Part model, mm, in its own coordinate system. A direction names the side the tool comes from. Round coordinates to 2 decimals unless told otherwise and drop trailing zeros. Loops run counter-clockwise (first coordinate to the right, second up) from the corner with the lowest first, then second, coordinate; pieces in that order, holes last.
from build123d import *

# Parameters (mm, degrees)
SKETCH1_R               = 50.00602605
SKETCH1_R_2             = 48.00602605
BOSS_EXTRUDE1_DEPTH     = 6.45
EXTRUDE_THIN1_START     = 4.55
SKETCH2_R               = 14.85
SKETCH2_R_2             = 11.85
EXTRUDE_THIN1_DEPTH     = 6.5
BOSS_EXTRUDE2_DEPTH     = 6.45
CUT_EXTRUDE1_DEPTH      = 7.45
CUT_EXTRUDE2_DEPTH      = 7.5
CUT_EXTRUDE3_DEPTH      = 1
CUT_EXTRUDE3_DEPTH_BACK = 7.5


with BuildPart() as part:
    # Sketch1 → Boss-Extrude1 (new body)
    with BuildSketch(Plane(origin=(0, 13.433589084, 0), x_dir=(-1, 0, 0), z_dir=(0, -1, 0))):
        with Locations((-83.776404782, 38.885320672)):
            Circle(SKETCH1_R)
        with Locations((-83.776404782, 38.885320672)):
            Circle(SKETCH1_R_2, mode=Mode.SUBTRACT)
    extrude(amount=BOSS_EXTRUDE1_DEPTH)



with BuildPart() as body_2:
    # Sketch2 → Extrude-Thin1 (new body)
    with BuildSketch(Plane(origin=(0, 17.983589084, 0), x_dir=(-1, 0, 0), z_dir=(0, -1, 0)).offset(EXTRUDE_THIN1_START)):
        with Locations((-208.585951979, 38.885320672)):
            Circle(SKETCH2_R)
        with Locations((-208.585951979, 38.885320672)):
            Circle(SKETCH2_R_2, mode=Mode.SUBTRACT)
    extrude(amount=EXTRUDE_THIN1_DEPTH)


with BuildPart() as part_1:
    add(part.part)

    add(body_2.part)  # Boss-Extrude2 merges body 2
    # Sketch3 → Boss-Extrude2 (add)
    with BuildSketch(Plane(origin=(0, 6.983589084, 0), x_dir=(-1, 0, 0), z_dir=(0, -1, 0))):
        with BuildLine():
            Line((-97.861971102, 86.866561409), (-212.768861048, 53.134031902))
            ThreePointArc((-212.768861048, 53.134031902), (-208.023442769, 53.724663089), (-203.336355819, 52.776477576))
            Line((-203.336355819, 52.776477576), (-113.385956141, 79.182679265))
            ThreePointArc((-113.385956141, 79.182679265), (-105.95919853, 83.701905803), (-97.861971102, 86.866561409))
        make_face()
        with BuildLine():
            Line((-113.385956141, -1.412037922), (-203.336355819, 24.994163767))
            ThreePointArc((-203.336355819, 24.994163767), (-208.023442769, 24.045978254), (-212.768861048, 24.636609441))
            Line((-212.768861048, 24.636609441), (-97.861971102, -9.095920066))
            ThreePointArc((-97.861971102, -9.095920066), (-105.95919853, -5.93126446), (-113.385956141, -1.412037922))
        make_face()
    extrude(amount=-BOSS_EXTRUDE2_DEPTH)

    # Sketch4 → Cut-Extrude1 (cut, through all)
    with BuildSketch(Plane(origin=(0, 6.983589084, 0), x_dir=(-1, 0, 0), z_dir=(0, -1, 0))):
        with BuildLine():
            Line((-113.385956141, 79.182679265), (-106.369670763, 81.242408265))
            ThreePointArc((-106.369670763, 81.242408265), (-131.782430832, 38.885320672), (-106.369670763, -3.471766922))
            Line((-106.369670763, -3.471766922), (-113.385956141, -1.412037922))
            ThreePointArc((-113.385956141, -1.412037922), (-133.782430832, 38.885320672), (-113.385956141, 79.182679265))
        make_face()
    extrude(amount=-CUT_EXTRUDE1_DEPTH, mode=Mode.SUBTRACT)

    # Sketch5 → Cut-Extrude2 (cut, through all)
    with BuildSketch(Plane(origin=(0, 6.933589084, 0), x_dir=(-1, 0, 0), z_dir=(0, -1, 0))):
        with BuildLine():
            Line((-203.336355819, 24.994163767), (-204.770657455, 25.415223133))
            Line((-204.770657455, 25.415223133), (-204.770657455, 52.35541821))
            Line((-204.770657455, 52.35541821), (-203.336355819, 52.776477576))
            ThreePointArc((-203.336355819, 52.776477576), (-193.735951979, 38.885320672), (-203.336355819, 24.994163767))
        make_face()
    extrude(amount=-CUT_EXTRUDE2_DEPTH, mode=Mode.SUBTRACT)

    # Sketch6 → Cut-Extrude3 (cut, two sides)
    with BuildSketch(Plane(origin=(0, 13.433589084, 0), x_dir=(1, 0, 0), z_dir=(0, 1, 0))) as cut_extrude3_sk:
        with BuildLine():
            Line((204.770657455, 25.415223133), (211.923828913, 27.515136963))
            ThreePointArc((211.923828913, 27.515136963), (208.3355607, 27.037966359), (204.770657455, 27.666317699))
            Line((204.770657455, 27.666317699), (204.770657455, 25.415223133))
        make_face()
        with BuildLine():
            Line((204.770657455, 50.104323644), (204.770657455, 52.35541821))
            Line((204.770657455, 52.35541821), (211.923828913, 50.25550438))
            ThreePointArc((211.923828913, 50.25550438), (208.3355607, 50.732674984), (204.770657455, 50.104323644))
        make_face()
    extrude(amount=CUT_EXTRUDE3_DEPTH, mode=Mode.SUBTRACT)
    extrude(cut_extrude3_sk.sketch, amount=-CUT_EXTRUDE3_DEPTH_BACK, mode=Mode.SUBTRACT)


solid = part_1.part
1) Drop flat-ended pins along their axis: pin 1 Ø1 at (x, y) = (74, 11) entering from +Z; pin 2 Ø1 at (y, z) = (11.5, -14.5) entering from -X; pin 3 Ø5 at (x, z) = (187, -60.5) entering from -Y. Give the stop position or say it passes through.
Values:
pin 1: stops at z = 10.25
pin 2: stops at x = 39.84
pin 3: stops at y = 6.98
2) Wall check: line 1 along Z through (x, y) = (85, 11.5); line 2 along Z through (x, y) = (94.5, 11); line 3 along X through (y, z) = (8.5, -37.5). Give the ranges that are in metal, low to high.
Values:
line 1: z = -88.88 to -86.88, 9.11 to 11.11
line 2: z = -87.73 to -85.68, 7.91 to 9.96
line 3: x = 33.79 to 35.79, 220.35 to 223.37
3) Tool access for faces 1 (the face through (143, 13.434, -72)), 2 (the face through (220.434, 10.229, -39.099)): list every direction of +Z, -Z, +X, -X, +Y, -Y with a clear straight run to the whole face (end or side of a thin tool).
Values:
face 1: +Z, -Z, +X, -X, +Y
face 2: +Y, -Y
4) Slice it at A-A, the plane y = 8. Give the cut face in (x, z).
Values:
outline: (97.86, -86.87) - (212.77, -53.13) arc R14.85 ccw to (212.77, -24.64) - (97.86, 9.1) arc R50.01 ccw (long way) to start; hole (106.37, -81.24) - (211.92, -50.26) arc R11.85 ccw to (211.92, -27.52) - (106.37, 3.47) arc R48.01 ccw (long way) to start
5) Slice it at C-C, the plane z = -75.5. Give the cut face in (x, y).
Values:
outline: (49.72, 6.98) - (52.73, 6.98) - (52.73, 13.43) - (49.72, 13.43) - close; (125.93, 6.98) - (136.58, 6.98) - (136.58, 13.43) - (125.93, 13.43) - close
6) Mould opens along X. For faces 3 (the face through (136.9, 6.984, -72.5)), 4 (the face through (154.511, 10.163, -70.236)), 5 (the face through (35.79, 10.25, -37.5)) say: released by +X, released by -X, zero draft, split by the parting line, or undercut.
Values:
face 3: zero draft
face 4: released by +X
face 5: undercut
7) Slice it at B-B, the plane x = 96. Give the cut face in (y, z), then the cut area to 3 significant figures.
Values:
outline: (6.98, -87.37) - (13.43, -87.37) - (13.43, -85.31) - (6.98, -85.31) - close; (6.98, 7.54) - (13.43, 7.54) - (13.43, 9.6) - (6.98, 9.6) - close
area: 26.6 mm2
